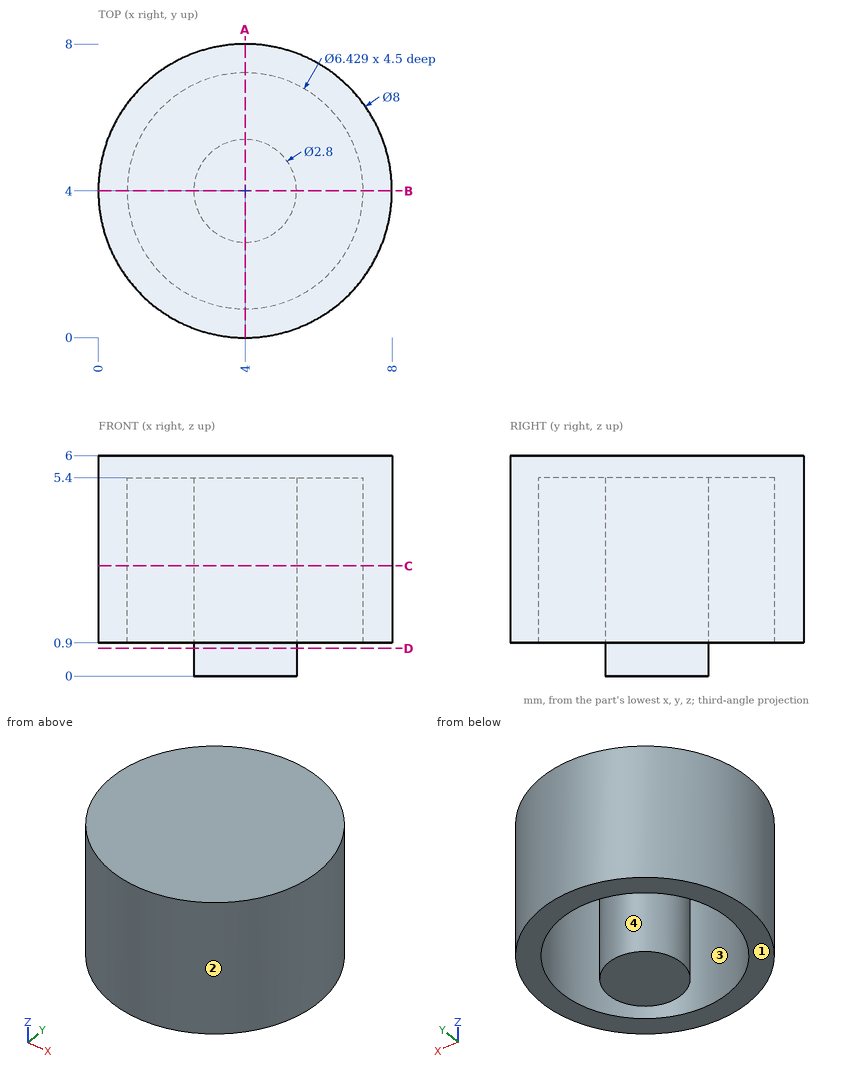
Drawing for the job (mm, zero at the part's lowest x, y, z). Round coordinates to 2 decimals unless told otherwise and drop trailing zeros. Loops run counter-clockwise (first coordinate to the right, second up) from the corner with the lowest first, then second, coordinate; pieces in that order, holes last. Notation, with made-up numbers: (55, -21) -> (84, -21) arc R32 cw to (84, 6) -> close; hole circle Ø4 at (-21.5, -34). An arc over 180 degrees is marked (long way). Answer in a Markdown table with one row per item.
Item 1: Saw through at C-C (z = 3). Write the cut outline in (x, y) (1 decimal).
Answers below:
| item | result |
|---|---|
| outline | circle Ø8 at (4, 4); circle Ø2.8 at (4, 4); hole circle Ø6.4 at (4, 4) |
Item 2: Mould opens along Y. For the marked faces 1, 2, 3 and 4 say: +Y half, -Y half, draft (parallel to the pull), parting line (faces both ways), or undercut.
Answers below:
| item | result |
|---|---|
| face 1 | draft |
| face 2 | parting line |
| face 3 | undercut |
| face 4 | undercut |
Item 3: Saw through at A-A (x = 4). Write the cut outline in (y, z) (1 decimal), and give its area (3 significant figures).
Answers below:
| item | result |
|---|---|
| outline | (0, 0.9) -> (0.8, 0.9) -> (0.8, 5.4) -> (2.6, 5.4) -> (2.6, 0) -> (5.4, 0) -> (5.4, 5.4) -> (7.2, 5.4) -> (7.2, 0.9) -> (8, 0.9) -> (8, 6) -> (0, 6) -> close |
| area | 27.0 mm² |
Item 4: Saw through at D-D (z = 0.75). Write the cut outline in (x, y).
Answers below:
| item | result |
|---|---|
| outline | circle Ø2.8 at (4, 4) |
Item 5: Drill centre lines: L1, parallel to X at y = 4, z = 3.1 (1 decimal); L2, parallel to X at y = 3, z = 4.2 (1 decimal). Where is each one in solid material? Low to high. Write a range as [from, to].
Answers below:
| item | result |
|---|---|
| L1 | x = [0, 0.8], [2.6, 5.4], [7.2, 8] |
| L2 | x = [0.1, 0.9], [3, 5], [7.1, 7.9] |
Item 6: Pin check, flat tips, straight feed: pin 1 (2 mm diameter, centred on x = 6.5, z = 1.5, fed in from +Y); pin 2 (1.5 mm diameter, centred on x = 6.5, z = 4.5, fed in from -Y). Stop position of each tip, or through.
Answers below:
| item | result |
|---|---|
| pin 1 | stops at y = 7.71 |
| pin 2 | stops at y = 0.4 |
